from build123d import *

# Parameters (mm, degrees)
RESSALTO_EXTRUS_O1_DEPTH = 2


with BuildPart() as part:
    # Esboço1 → Ressalto-extrusão1 (new body)
    with BuildSketch(Plane(origin=(0, 0, 0), x_dir=(1, 0, 0), z_dir=(0, 1, 0))):
        with BuildLine():
            Line((-23, 14.5), (23, 14.5))
            ThreePointArc((23, 14.5), (24.414213562, 13.914213562), (25, 12.5))
            Line((25, 12.5), (25, -14.5))
            Line((25, -14.5), (-25, -14.5))
            Line((-25, -14.5), (-25, 12.5))
            ThreePointArc((-25, 12.5), (-24.414213562, 13.914213562), (-23, 14.5))
        make_face()
        with BuildLine():
            Line((-10, 5.5), (-10, -8.5))
            ThreePointArc((-10, -8.5), (-11, -9.5), (-12, -8.5))
            Line((-12, -8.5), (-12, 5.5))
            ThreePointArc((-12, 5.5), (-11, 6.5), (-10, 5.5))
        make_face(mode=Mode.SUBTRACT)
        with BuildLine():
            Line((10, 5.5), (10, -8.5))
            ThreePointArc((10, -8.5), (11, -9.5), (12, -8.5))
            Line((12, -8.5), (12, 5.5))
            ThreePointArc((12, 5.5), (11, 6.5), (10, 5.5))
        make_face(mode=Mode.SUBTRACT)
    extrude(amount=RESSALTO_EXTRUS_O1_DEPTH)


solid = part.part
Design review of the part built by this model. Coordinates are the model's own, in mm. A direction names the side the tool comes from. Give positions to 0.01 mm unless a question says otherwise; leave off trailing zeros. Loops run counter-clockwise (first coordinate to the right, second up) from the corner with the lowest first, then second, coordinate; pieces in that order, holes last. Notation, with made-up numbers: (25, 63) - (41, 63) arc R23 cw to (41, 75) - close; hole circle Ø3 at (5.5, -22.5). An arc over 180 degrees is marked (long way). Use CSV: the item, a comma, the result in double quotes. Start each with the question number.
1. Machinability: for faces 5 (the flat face through (-25, 1, 1)), 6 (the cylindrical face through (-11, 1, -6.5)), which of the approach directions +Z, -Z, +X, -X, +Y, -Y give a long, thin tool a straight path to every point of the face, cutting with its end or side? Answer none if there is none.
2. Draft analysis for pull direction Z (two halves, no side actions). For faces 1 (the flat face through (-10, 1, 1)), 2 (the cylindrical face through (-24.43, 0.99, -13.9)), 3 (the cylindrical face through (11, 1, -6.5)), 4 (the flat face through (0, 0, 0)), state which applies: released by +Z, released by -Z, zero draft, split by the parting line, or undercut.
3. Add section A-A (z = 3.5). State the section outline as (x, y) points, plus the area to 3 significant figures.
4. Add section C-C (y = 0.85). State the section outline as (x, z) points.
5. Wall thickness on L1, parallel to X at y = 0.35, z = 6.75: over which ranges is the line inside the solid? List them lowest first.
6. Add section B-B (x = 11). State the section outline as (y, z) points, plus the area to 3 significant figures.
Results found:
1,face 5,"+Z, -Z, -X, +Y, -Y"
1,face 6,"+Y, -Y"
2,face 1,"undercut"
2,face 2,"released by -Z"
2,face 3,"undercut"
2,face 4,"zero draft"
3,outline,"(-25, 0) - (-12, 0) - (-12, 2) - (-25, 2) - close; (-10, 0) - (10, 0) - (10, 2) - (-10, 2) - close; (12, 0) - (25, 0) - (25, 2) - (12, 2) - close"
3,area,"92.0 mm²"
4,outline,"(-25, -12.5) arc R2 ccw to (-23, -14.5) - (23, -14.5) arc R2 ccw to (25, -12.5) - (25, 14.5) - (-25, 14.5) - close; hole (-12, -5.5) arc R1 ccw to (-10, -5.5) - (-10, 8.5) arc R1 ccw to (-12, 8.5) - close; hole (10, -5.5) arc R1 ccw to (12, -5.5) - (12, 8.5) arc R1 ccw to (10, 8.5) - close"
5,L1,"x = -25 to -12, -10 to 10, 12 to 25"
6,outline,"(0, -14.5) - (2, -14.5) - (2, -6.5) - (0, -6.5) - close; (0, 9.5) - (2, 9.5) - (2, 14.5) - (0, 14.5) - close"
6,area,"26.0 mm²"
